```python
from build123d import *

# Parameters (mm, degrees)
SKETCH1_W           = 500
SKETCH1_H           = 150
SKETCH1_R           = 9.3
SKETCH1_R_2         = 3
SKETCH1_R_3         = 4
BOSS_EXTRUDE1_DEPTH = 7
CUT_EXTRUDE1_DEPTH  = 7
FILLET2_R           = 3


with BuildPart() as part:
    # Sketch1 → Boss-Extrude1 (new body)
    with BuildSketch(Plane.XY):
        with Locations((200, 0)):
            Rectangle(SKETCH1_W, SKETCH1_H)
        Circle(SKETCH1_R, mode=Mode.SUBTRACT)
        with BuildLine():
            ThreePointArc((303.793920425, 21.250000148), (340.59999997, 42.5), (377.406079545, 21.250000201))
            ThreePointArc((377.406079545, 21.250000201), (375.758965412, 15.102885723), (369.61185099, 16.750000063))
            ThreePointArc((369.61185099, 16.750000063), (340.600001147, 33.5), (311.588150157, 16.750002051))
            ThreePointArc((311.588150157, 16.750002051), (305.441035607, 15.102885134), (303.793920425, 21.250000148))
        make_face(mode=Mode.SUBTRACT)
        with Locations((377.305181399, -9.835123714)):
            Circle(SKETCH1_R_2, mode=Mode.SUBTRACT)
        with Locations((340.6, 0)):
            Circle(SKETCH1_R_3, mode=Mode.SUBTRACT)
    extrude(amount=BOSS_EXTRUDE1_DEPTH)

    # Sketch3 → Cut-Extrude1 (cut)
    with BuildSketch(Plane.XY.offset(7)):
        with BuildLine():
            Line((69.562794416, 55), (-50, 55))
            Line((-50, 55), (-50, -75))
            Line((-50, -75), (450, -75))
            Line((450, -75), (450, 55))
            Line((450, 55), (340.6, 55))
            ThreePointArc((340.6, 55), (379.490872965, 38.890872965), (395.6, 0))
            ThreePointArc((395.6, 0), (394.762205793, -9.563235), (392.274346776, -18.835123714))
            ThreePointArc((392.274346776, -18.835123714), (329.562623749, -53.881131442), (285.681879129, 3))
            Line((285.681879129, 3), (30.896152423, 3))
            Line((30.896152423, 3), (6.425, -11.128426439))
            ThreePointArc((6.425, -11.128426439), (-11.128426439, -6.425), (-6.425, 11.128426439))
            Line((-6.425, 11.128426439), (69.562794416, 55))
        make_face()
        with BuildLine():
            Line((328.4653389, 3), (285.681879129, 3))
            ThreePointArc((285.681879129, 3), (329.562623749, -53.881131442), (392.274346776, -18.835123714))
            Line((392.274346776, -18.835123714), (371.498146439, -18.835123714))
            Line((371.498146439, -18.835123714), (350.968741122, -6.981347115))
            ThreePointArc((350.968741122, -6.981347115), (335.531820751, -11.426441226), (328.4653389, 3))
        make_face()
        Polygon((-50, 75), (-50, 55), (69.562794416, 55), (340.6, 55), (450, 55), (450, 75), align=None)
    extrude(amount=-CUT_EXTRUDE1_DEPTH, mode=Mode.SUBTRACT)

    # Fillet2
    fillet2_edges = [part.edges().sort_by_distance(p)[0] for p in [
        (69.562794416, 55, 3.5),
        (30.896152423, 3, 3.5),
        (328.4653389, 3, 3.5),
        (350.968741122, -6.981347115, 3.5),
    ]]
    fillet(fillet2_edges, radius=FILLET2_R)


solid = part.part
```
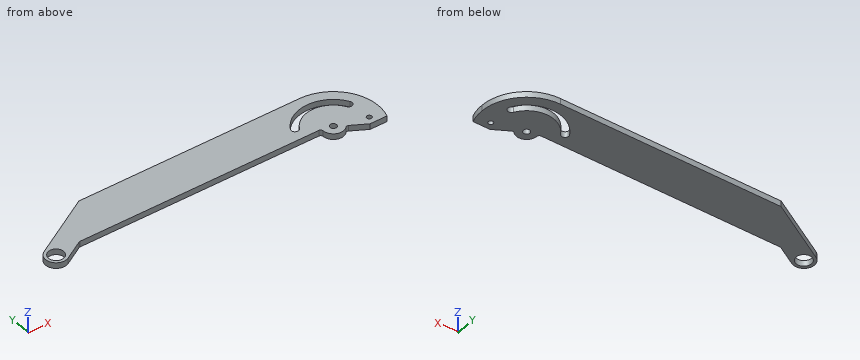
Can you work these out from the model? Positions are in its coordinate system, mm. Give positions to 0.01 mm unless a question says otherwise; leave off trailing zeros. Write each loop counter-clockwise with the first axis right and the second up, starting at its lowest first coordinate (ties: lowest second). Pieces come first, ordered by that corner, then holes. Notation, with made-up numbers: (-26, 27) - (-15, 27) arc R20 cw to (-15, 46) - close; hole circle Ø7 at (-13.5, 58.25). An arc over 180 degrees is marked (long way). Write item = value, one per line. Start each with the question number.
1. Imagine slicing it at A-A (z = 3.75). Please give me the cut outline in (x, y) (3 decimals), and give its area (3 significant figures).
2. Imagine slicing it at B-B (x = 0). Please give me the cut outline in (y, z), and give its area (3 significant figures).
3. Please list where these lines run through material, in increasing order: line 1 (X direction, y = -5, z = 5.75); line 2 (Y direction, x = 83.5, z = 5.25); line 3 (X direction, y = 39, z = 5.5).
4. For pin 1 (2 mm diameter, centred on x = 54.5, z = 5, fed in from -Y); pin 2 (2 mm diameter, centred on y = 37.5, z = 1.5, fed in from +X), each with a flat end and sliding along its axis, tell me the tip position at first contact or that it passes through.
5. Imagine slicing it at C-C (x = 258). Please give me the cut outline in (y, z).
Worked answers:
q1.outline = (-6.425, 11.128) arc R12.85 ccw to (6.425, -11.128) - (30.2, 2.598) arc R3 cw to (31.7, 3) - (325.1, 3) arc R3 cw to (328.1, 0) arc R12.5 ccw to (349.527, -8.75) arc R3 cw to (353.169, -8.252) - (371.498, -18.835) - (392.274, -18.835) arc R55 ccw to (340.6, 55) - (70.367, 55) arc R3 ccw to (68.867, 54.598) - close; hole circle Ø18.6 at (0, 0); hole (303.794, 21.25) arc R4.5 ccw to (311.588, 16.75) arc R33.5 cw to (369.612, 16.75) arc R4.5 ccw to (377.406, 21.25) arc R42.5 ccw to start; hole circle Ø8 at (340.6, 0); hole circle Ø6 at (377.305, -9.835)
q1.area = 19,100 mm2
q2.outline = (-12.85, 0) - (-9.3, 0) - (-9.3, 7) - (-12.85, 7) - close; (9.3, 0) - (14.84, 0) - (14.84, 7) - (9.3, 7) - close
q2.area = 63.6 mm2
q3.line_1 = -11.84 to -7.84, 7.84 to 17.04, 329.14 to 395.37
q3.line_2 = 3 to 55
q3.line_3 = 41.85 to 323.71, 357.49 to 379.38
q4.pin_1 = 3
q4.pin_2 = 381.74
q5.outline = (3, 0) - (55, 0) - (55, 7) - (3, 7) - close
